CAD build for the part. Positions are in the model's coordinates, mm. A direction names the side the tool comes from. Round coordinates to 2 decimals unless told otherwise and drop trailing zeros. Write each loop counter-clockwise with the first axis right and the second up, starting at its lowest first coordinate (ties: lowest second). Pieces come first, ordered by that corner, then holes. Notation, with made-up numbers: (-27, 19.5) - (-22, 19.5) arc R6 cw to (-22, 28.5) - close; hole circle Ø11 at (80, -28.5). An arc over 180 degrees is marked (long way). Put each result on its own line as item: value. Start each with the question number.
Item 1: 3-axis set-ups, long thin cutter, end or side, ignore diameter. For faces 5 (the flat face through (-112.085, -46.669, 216.935)), 6 (the cylindrical face through (12.173, -46.669, 269.16)), 7 (the flat face through (-58.09, -46.67, 228.28)): which of +Z, -Z, +X, -X, +Y, -Y reach the whole face in a straight line?
Item 2: Cut at B-B (x = 33). Give the cut face in (y, z).
Item 3: Drill centre lines: line 1 (Z direction, x = 117, y = -44.75); line 2 (X direction, y = -45.25, z = 185.5); line 3 (Z direction, x = -18, y = -46). Where is each one in solid material? Low to high. Write a range as from..to.
Item 4: Mould opens along X. For faces 1 (the cylindrical face through (6.75, -46.67, 248.93)), 2 (the flat face through (-133.35, -47, 189)), 3 (the flat face through (2, -43.45, 199)), 4 (the flat face through (133.35, -47, 172)) say: released by +X, released by -X, zero draft, split by the parting line, or undercut.
Item 5: Cut at C-C (z = 229). Give the cut face in (x, y).
Item 6: Cut at A-A (y = -45.75). Give the cut face in (x, z), and give its area (3 significant figures).
Item 7: Pin check, flat tips, straight feed: pin 1 Ø8 at (x, z) = (-62.5, 234) entering from +Y; pin 2 Ø2 at (y, z) = (-47, 237.5) entering from +X. Stop position of each tip, or through.
```python
from build123d import *

# Parameters (mm, degrees)
PAD005_DEPTH    = 6.35
SKETCH014_W     = 3.141259
SKETCH014_H     = 4.397751
PAD011_DEPTH    = 6.35
SKETCH015_W     = 9.97554
SKETCH015_H     = 9.591858
PAD012_DEPTH    = 6.35
POCKET001_DEPTH = 6.35
PAD016_DEPTH    = 6.35


with BuildPart() as part:
    # Sketch006 (on Face1 of ShapeBinder007) → Pad005 (new body)
    with BuildSketch(Plane.XZ.offset(49.8)):
        with BuildLine():
            Line((133.35, 169.55), (-133.35, 169.55))
            Line((-133.35, 169.55), (-133.35, 209.55))
            Line((-10.630146, 252.168791), (-133.35, 209.55))
            ThreePointArc((-10.630146, 252.168791), (6.989684, 249.06987), (12.862348, 265.968791))
            Line((12.862348, 265.968791), (22.18289, 269.591979))
            Line((133.35, 174.55), (22.18289, 269.591979))
            Line((133.35, 169.55), (133.35, 174.55))
        make_face()
    extrude(amount=-PAD005_DEPTH)

    # Sketch014 (on Face8 of Pad005) → Pad011 (join)
    with BuildSketch(Plane.XZ.offset(49.8)):
        with Locations((-75.779384, 200.48986)):
            Rectangle(SKETCH014_W, SKETCH014_H)
    extrude(amount=-PAD011_DEPTH)

    # Sketch015 (on Face8 of Pad011) → Pad012 (join)
    with BuildSketch(Plane.XZ.offset(49.8)):
        with Locations((45.684311, 201.652512)):
            Rectangle(SKETCH015_W, SKETCH015_H)
    extrude(amount=-PAD012_DEPTH)

    # Sketch050 (on Face8 of Pad012) → Pocket001 (cut)
    with BuildSketch(Plane.XZ.offset(49.8)):
        with BuildLine():
            ThreePointArc((-83.081656, 223.304195), (-87.155196, 224.622491), (-91.406711, 224.116284))
            Line((-91.406711, 224.116284), (-93.047035, 228.83956))
            Line((-93.047035, 228.83956), (-31.459503, 250.228))
            Line((-31.459503, 250.228), (-29.819179, 245.504724))
            ThreePointArc((-29.819179, 245.504724), (-33.469298, 243.26681), (-35.848895, 239.707435))
            ThreePointArc((-41.878611, 233.910146), (-38.228492, 236.14806), (-35.848895, 239.707435))
            Line((-41.878611, 233.910146), (-74.756601, 222.492106))
            ThreePointArc((-83.081656, 223.304195), (-79.008116, 221.985899), (-74.756601, 222.492106))
        make_face()
    extrude(amount=-POCKET001_DEPTH, mode=Mode.SUBTRACT)

    # Sketch051 (on Face4 of Pocket001) → Pad016 (join)
    with BuildSketch(Plane.XZ.offset(49.8)):
        with BuildLine():
            ThreePointArc((12.862348, 265.968791), (12.157812, 269.203321), (10.647338, 272.149))
            Line((10.647338, 272.149), (12.307973, 273.263581))
            ThreePointArc((18.295876, 272.91517), (15.360549, 274.096912), (12.307973, 273.263581))
            Line((18.295876, 272.91517), (22.18289, 269.591979))
            Line((22.18289, 269.591979), (12.862348, 265.968791))
        make_face()
    extrude(amount=-PAD016_DEPTH)


solid = part.part
```
Output values:
1. face 5: +Z, -X, +Y, -Y
1. face 6: -X, +Y, -Y
1. face 7: +Z, +Y, -Y
2. outline: (-49.8, 169.55) - (-43.45, 169.55) - (-43.45, 260.34) - (-49.8, 260.34) - close
3. line 1: 169.55..188.53
3. line 2: -133.35..120.54
3. line 3: 169.55..249.61
4. face 1: undercut
4. face 2: released by -X
4. face 3: zero draft
4. face 4: released by +X
5. outline: (-56.02, -49.8) - (69.66, -49.8) - (69.66, -43.45) - (-56.02, -43.45) - close
6. outline: (-133.35, 169.55) - (133.35, 169.55) - (133.35, 174.55) - (18.3, 272.92) arc R4.96 ccw to (12.31, 273.26) - (10.65, 272.15) arc R12.8 cw to (12.86, 265.97) arc R13.8 cw to (-10.63, 252.17) - (-29.82, 245.5) arc R10 ccw to (-35.85, 239.71) arc R10 cw to (-41.88, 233.91) - (-74.76, 222.49) arc R10 cw to (-83.08, 223.3) arc R10 ccw to (-91.41, 224.12) - (-133.35, 209.55) - close
6. area: 15,800 mm2
7. pin 1: through
7. pin 2: x = 60.89
